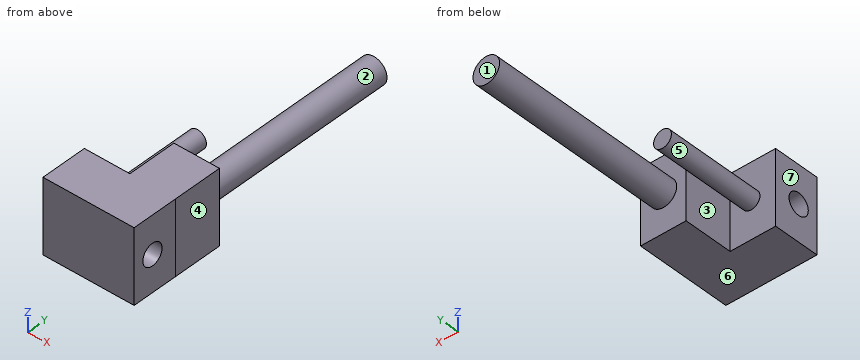
Autodesk Inventor part; units mm, degrees
ref_plane "YZ Plane" through (0, 0, 0) normal (1, 0, 0) x (0, 1, 0)
ref_plane "XZ Plane" through (0, 0, 0) normal (0, 1, 0) x (-1, 0, 0)
ref_plane "XY Plane" through (0, 0, 0) normal (0, 0, 1) x (1, 0, 0)
sketch "스케치1" plane through (0, 0, 0) normal (0, 0, 1) x (1, 0, 0)
  line L0 (36.9529, -18.7887) -> (-36.9529, -18.7887)
  line L1 (-36.9529, -18.7887) -> (-36.9529, 18.7887)
  line L2 (-36.9529, 18.7887) -> (36.9529, 18.7887)
  line L3 (36.9529, 18.7887) -> (36.9529, -18.7887)
  line L4 (36.9529, -18.7887) -> (-36.9529, 18.7887) construction
  line L5 (-36.9529, -18.7887) -> (36.9529, 18.7887) construction
  point P0 (0, 0)
extrude "돌출1" add sketch "스케치1" along normal blind 60
sketch "스케치2" plane through (-36.9529, 18.7887, 0) normal (0, 1, 0) x (1, 0, 0)
  line L0 (73.9059, 0) -> (73.9059, -60)
  line L1 (36.9529, 0) -> (73.9059, 0)
  line L2 (73.9059, 0) -> (73.9059, -60)
  line L3 (73.9059, -60) -> (36.9529, -60)
  line L4 (36.9529, -60) -> (36.9529, 0)
  circle A0 centre (55.4294, -30) radius 7.9669
extrude "돌출2" add sketch "스케치2" along normal blind 40 contours L0 L3 L4 L1 | A0
sketch "스케치3" plane through (-36.9529, 18.7887, 60) normal (0, 1, 0) x (1, 0, 0)
  circle A0 centre (19.9645, 29.7419) radius 7.2214
  point P0 (36.9529, 60)
extrude "돌출3" add sketch "스케치3" along normal blind 80.5
sketch "스케치4" plane through (-36.9529, 58.7887, 0) normal (0, 1, 0) x (1, 0, 0)
  circle A0 centre (55.3783, -30.6807) radius 10.7619
  point P0 (36.9529, 0)
extrude "돌출4" add sketch "스케치4" along normal blind 161
sketch "스케치5" plane through (-36.9529, -18.7887, 0) normal (-1, 0, 0) x (0, 0, 1)
  circle A0 centre (29.4129, 16.6757) radius 8.7461
  point P0 (0, 18.7887)
extrude "돌출5" cut sketch "스케치5" against normal blind 80.5
properties part number "240503_3Dsketch01"
Geometry: final body of the model. Coordinates: model frame, mm. Face numbers are marked on the shaded views. A direction names the side the tool comes from. Round coordinates to 2 decimals unless told otherwise and drop trailing zeros. Order: outer loops, then holes, each group sorted by start corner. A loop starts at its lowest first (then second) coordinate and runs counter-clockwise, first axis right, second up. Notation, with made-up numbers: (-23.5, 64) - (-12.5, 64) arc R10 ccw to (-12.5, 73) - close; hole circle Ø11 at (-27, 7.5). An arc over 180 degrees is marked (long way). Write each question's results on one line, items separated by ' | '.
Item 1: Section B-B, the plane x = 12. Return the cut outline in (y, z), and give its area (3 significant figures).
Completed:
outline: (-18.79, 0) - (58.79, 0) - (58.79, 22.05) - (219.79, 22.05) - (219.79, 39.31) - (58.79, 39.31) - (58.79, 60) - (-18.79, 60) - close; hole circle Ø17.49 at (-2.11, 29.41) | area: 7,190 mm^2
Item 2: Reachability of the marked faces 1, 2 and 3 from +Z, -Z, +X, -X, +Y, -Y: full face, straight path, thin tool, end or side. Return the list, or none.
Completed:
face 1: +Z, -Z, +X, -X, +Y | face 2: +Y | face 3: +Z, -Z, +Y
Item 3: Material intervals for line 1 along Y through (x, z) = (22, 49); line 2 along Y through (x, z) = (-5, 7); line 3 along X through (y, z) = (35.5, 3.5), sorted ascending. Write a range as [from, to].
Completed:
line 1: [-18.79, 58.79] | line 2: [-18.79, 18.79] | line 3: [0, 36.95]
Item 4: Section D-D, the plane y = 23. Return the cut outline in (x, z).
Completed:
outline: circle Ø14.44 at (-16.99, 30.26); (0, 0) - (36.95, 0) - (36.95, 60) - (0, 60) - close
Item 5: First-contact query: pin 1 Ø1.5 at (x, z) = (-9, 51) entering from +Y; pin 2 Ø6 at (y, z) = (51.5, 38.5) entering from -X; pin 3 Ø1.5 at (x, y) = (12, 189) entering from +Z. Flat tips, straight axial feed; report the tip coordinate or a pass-through.
Completed:
pin 1: y = 18.79 | pin 2: x = -21.96 | pin 3: z = 39.82
Item 6: Mould query, pull axis X, two halves, no side actions, for the marked faces 4, 5, 6 and 7. Classes: pulls with the +X half, pulls with the -X half, needs draft (parallel to the pull), parting line crosses it, or undercut.
Completed:
face 4: pulls with the +X half | face 5: undercut | face 6: needs draft | face 7: pulls with the -X half
